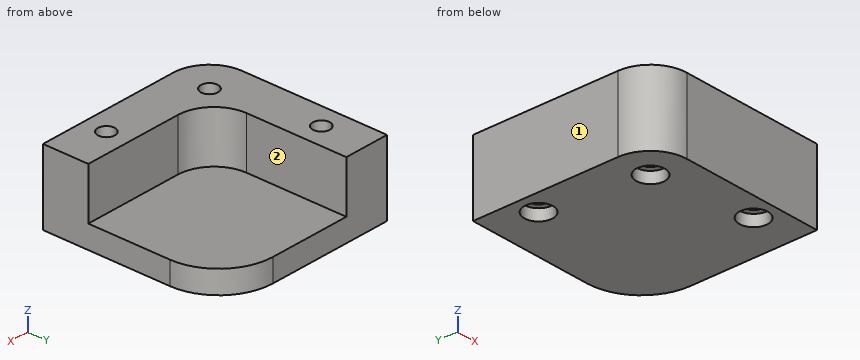
from build123d import *

# Parameters (mm, degrees)
F0_W     = 25.4
F0_H     = 25.4
F1_DEPTH = 3.175
F3_DEPTH = 10.31875
F4_R     = 5.08
F5_R     = 7.62
F6_R     = 1.190625
F7_DEPTH = 10.31975
F8_R     = 1.984375
F9_DEPTH = 1.5875


with BuildPart() as f1:
    # F0 (on Top) → F1 (new body)
    with BuildSketch(Plane.XY):
        with Locations((14.847793, 12.7)):
            Rectangle(F0_W, F0_H)
    extrude(amount=F1_DEPTH)

    # F2 (on Top) → F3 (join)
    with BuildSketch(Plane.XY):
        Polygon((2.147793, 6.35), (2.147793, 0), (8.497793, 0), (27.547793, 0), (27.547793, 6.35), (8.497793, 6.35), (8.497793, 25.4), (2.147793, 25.4), align=None)
    extrude(amount=F3_DEPTH)

    # F4
    f4_edges = [f1.edges().sort_by_distance(p)[0] for p in [
        (8.497793, 6.35, 6.746875),
        (2.147793, 0, 5.159375),
    ]]
    fillet(f4_edges, radius=F4_R)

    # F5
    f5_edges = [f1.edges().sort_by_distance(p)[0] for p in [
        (27.547793, 25.4, 1.5875),
    ]]
    fillet(f5_edges, radius=F5_R)

    # F6 (on face) → F7 (cut, through all)
    with BuildSketch(Plane.XY.offset(10.31875)):
        with Locations((7.227793, 5.08)):
            Circle(F6_R)
        with Locations((5.322793, 19.05)):
            Circle(F6_R)
        with Locations((21.197793, 3.175)):
            Circle(F6_R)
    extrude(amount=-F7_DEPTH, mode=Mode.SUBTRACT)

    # F8 (on face) → F9 (cut)
    with BuildSketch(Plane(origin=(0, 0, 0), x_dir=(1, 0, 0), z_dir=(0, 0, -1))):
        with Locations((7.227793, -5.08)):
            Circle(F8_R)
        with Locations((21.197793, -3.175)):
            Circle(F8_R)
        with Locations((5.322793, -19.05)):
            Circle(F8_R)
    extrude(amount=-F9_DEPTH, mode=Mode.SUBTRACT)


solid = f1.part
Check sheet for the modelled part. Datum: model origin and axes. Units: mm. Face numbers are marked on the shaded views. A direction names the side the tool comes from. Round coordinates to 2 decimals unless told otherwise and drop trailing zeros. Order: outer loops, then holes, each group sorted by start corner. A loop starts at its lowest first (then second) coordinate and runs counter-clockwise, first axis right, second up.
Q1. Cross-section at C-C, the plane x = 16. Enter the section's corners in (y, z) (3 decimals).
Filled sheet:
outline: (0, 0) - (25.4, 0) - (25.4, 3.175) - (6.35, 3.175) - (6.35, 10.319) - (0, 10.319) - close
Q2. Cross-section at B-B, the plane z = 2.25. Enter the section's corners in (x, y) (3 decimals), plus the area to 3 significant figures.
Filled sheet:
outline: (2.148, 5.08) arc R5.08 ccw to (7.228, 0) - (27.548, 0) - (27.548, 17.78) arc R7.62 ccw to (19.928, 25.4) - (2.148, 25.4) - close; hole circle Ø2.381 at (5.323, 19.05); hole circle Ø2.381 at (7.228, 5.08); hole circle Ø2.381 at (21.198, 3.175)
area: 614 mm2
Q3. Depth check by flat-ended pin: P1, Ø1.5, axis at x = 19, z = 4, coming from the +Y side; P2, Ø2.5, axis at x = 21.2, y = 3.18, coming from the -Z side; P3, Ø5.5, axis at y = 19.5, z = 8.5, coming from the +X side. Enter the tip coordinate at first touch or a pass-through.
Filled sheet:
P1: stops at y = 6.35
P2: stops at z = 1.59
P3: stops at x = 8.5
Q4. Cross-section at A-A, the plane y = 19.05. Enter the section's corners in (x, z) (1 decimal), plus the area to 3 significant figures.
Filled sheet:
outline: (2.1, 0) - (3.3, 0) - (3.3, 1.6) - (4.1, 1.6) - (4.1, 10.3) - (2.1, 10.3) - close; (6.5, 1.6) - (7.3, 1.6) - (7.3, 0) - (27.4, 0) - (27.4, 3.2) - (8.5, 3.2) - (8.5, 10.3) - (6.5, 10.3) - close
area: 98.6 mm2
Q5. Scan lines: L1, parallel to X at y = 13.75, z = 7; L2, parallel to Z at x = 14.5, y = 21.25 (3 decimals); L3, parallel to Y at x = 24.5, z = 7.75. Record each from-to range of solid material in increasing order.
Filled sheet:
L1: x = 2.15 to 8.5
L2: z = 0 to 3.175
L3: y = 0 to 6.35
Q6. Set-up check for the marked faces 1 and 2: record each of +Z, -Z, +X, -X, +Y, -Y from which the full face is reachable in a straight line by a thin tool's end or side.
Filled sheet:
face 1: +Z, -Z, -X, +Y, -Y
face 2: +Z, +X, +Y
